```python
from build123d import *

# Parameters (mm, degrees)
EXTRUDE_1_DEPTH     = 50.5
EXTRUDE_2_DEPTH     = 4
CHAMFER_1_SIZE      = 10
SKETCH_3_R          = 4
CUT_EXTRUDE_1_DEPTH = 10
SKETCH_4_R          = 4
CUT_EXTRUDE_2_DEPTH = 10
SKETCH_5_R          = 2.5
CUT_EXTRUDE_3_DEPTH = 10


with BuildPart() as part:
    # 草图1 → 凸台-拉伸1 (new body)
    with BuildSketch(Plane.XY):
        Polygon((-12.426406871, 30), (-30, 12.426406871), (-30, -12.426406871), (-12.426406871, -30), (-12.426406871, -32.828427125), (-32, -13.254833996), (-32, 13.254833996), (-12.426406871, 32.828427125), align=None)
    extrude(amount=EXTRUDE_1_DEPTH)

    # 草图2 → 凸台-拉伸2 (add)
    with BuildSketch(Plane(origin=(0, 0, 0), x_dir=(-1, 0, 0), z_dir=(0, 0, -1))):
        Polygon((12.426406871, 30), (12.426406871, 40), (47.426406871, 40), (47.426406871, -40), (12.426406871, -40), (12.426406871, -30), (30, -12.426406871), (30, 12.426406871), align=None)
    extrude(amount=EXTRUDE_2_DEPTH)

    # 倒角1
    chamfer_1_edges = [part.edges().sort_by_distance(p)[0] for p in [
        (-47.426406871, -40, -2),
        (-47.426406871, 40, -2),
    ]]
    chamfer(chamfer_1_edges, length=CHAMFER_1_SIZE)

    # 草图3 → 切除-拉伸1 (cut)
    with BuildSketch(Plane(origin=(-22.627416998, 22.627416998, 0), x_dir=(0, 0, 1), z_dir=(-0.707106781, 0.707106781, 0))):
        with Locations((40.5, 0.585786438)):
            Circle(SKETCH_3_R)
        with Locations((24.5, 0.585786438)):
            Circle(SKETCH_3_R)
    cut_extrude_1 = extrude(amount=-CUT_EXTRUDE_1_DEPTH, mode=Mode.SUBTRACT)

    # 草图4 → 切除-拉伸2 (cut)
    with BuildSketch(Plane.ZY.offset(32)):
        with Locations((32.5, 0)):
            Circle(SKETCH_4_R)
    extrude(amount=-CUT_EXTRUDE_2_DEPTH, mode=Mode.SUBTRACT)

    # 镜向1: 切除-拉伸1 across plane
    add(cut_extrude_1.mirror(Plane.ZX), mode=Mode.SUBTRACT)

    # 草图5 → 切除-拉伸3 (cut)
    with BuildSketch(Plane.XY):
        with Locations((-38, 30)):
            Circle(SKETCH_5_R)
        with Locations((-38, -30)):
            Circle(SKETCH_5_R)
    extrude(amount=-CUT_EXTRUDE_3_DEPTH, mode=Mode.SUBTRACT)


solid = part.part
```
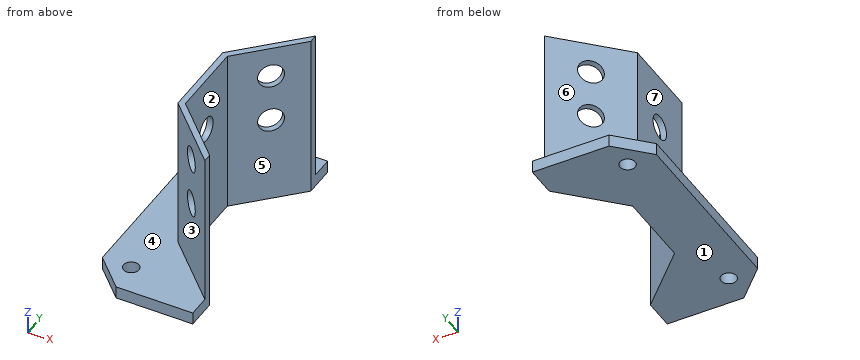
Model file for the job. Use its own axes, mm. Face numbers are marked on the shaded views. A direction names the side the tool comes from. Give positions to 0.01 mm unless a question says otherwise; leave off trailing zeros. Loops run counter-clockwise (first coordinate to the right, second up) from the corner with the lowest first, then second, coordinate; pieces in that order, holes last. Notation, with made-up numbers: (46, 9.25) -> (58, 9.25) arc R13 cw to (58, 13.25) -> close; hole circle Ø2 at (5.25, -13.5). An arc over 180 degrees is marked (long way). Write each question's results on one line, items separated by ' | '.
(1) Flat gauge pins, fed straight in: pin 1 Ø12 at (x, z) = (-24.5, 40) entering from -Y; pin 2 Ø13.5 at (y, z) = (-6, 30) entering from -X; pin 3 Ø6.5 at (x, y) = (-38, -30) entering from +Z. Where does each tip first touch, or does it go through?
Geometry results:
pin 1: stops at y = -26.75 | pin 2: stops at x = -32 | pin 3: stops at z = 0
(2) Pull direction Y, two halves, no side cores. Call the marked faces 1, 2 and 3: released by +Y, released by -Y, zero draft, split by the parting line, or undercut.
Geometry results:
face 1: zero draft | face 2: undercut | face 3: released by -Y
(3) Cut at C-C on z = 19. List the corners of the cut face in (x, y), and give its area (3 significant figures).
Geometry results:
outline: (-32, -13.25) -> (-12.43, -32.83) -> (-12.43, -30) -> (-30, -12.43) -> (-30, 12.43) -> (-12.43, 30) -> (-12.43, 32.83) -> (-32, 13.25) -> close | area: 156 mm²
(4) Cut at A-A on y = 0. List the corners of the cut face in (x, z).
Geometry results:
outline: (-47.43, -4) -> (-30, -4) -> (-30, 28.5) -> (-32, 28.5) -> (-32, 0) -> (-47.43, 0) -> close; (-32, 36.5) -> (-30, 36.5) -> (-30, 50.5) -> (-32, 50.5) -> close
(5) Cut at B-B on x = -38.5. List the corners of the cut face in (y, z), and give its area (3 significant figures).
Geometry results:
outline: (-38.93, -4) -> (-32.45, -4) -> (-32.45, 0) -> (-38.93, 0) -> close; (-27.55, -4) -> (27.55, -4) -> (27.55, 0) -> (-27.55, 0) -> close; (32.45, -4) -> (38.93, -4) -> (38.93, 0) -> (32.45, 0) -> close | area: 272 mm²
(6) Cut at D-D on z = 35.5. List the corners of the cut face in (x, y), and give its area (3 significant figures).
Geometry results:
outline: (-32, -13.25) -> (-12.43, -32.83) -> (-12.43, -30) -> (-30, -12.43) -> (-30, -2.65) -> (-32, -2.65) -> close; (-32, 2.65) -> (-30, 2.65) -> (-30, 12.43) -> (-12.43, 30) -> (-12.43, 32.83) -> (-32, 13.25) -> close | area: 146 mm²
(7) Probe line 1 along Y through (x, z) = (-38, -1); line 2 along Z through (x, y) = (-34.5, 8); line 3 along Y through (x, z) = (-31, 32). List the from-to ranges inside material, lowest first.
Geometry results:
line 1: y = -39.43 to -32.5, -27.5 to 27.5, 32.5 to 39.43 | line 2: z = -4 to 0 | line 3: y = -14.25 to -3.97, 3.97 to 14.25
(8) Tool access for the marked faces 4, 5, 6 and 7: list every direction of +Z, -Z, +X, -X, +Y, -Y with a clear straight run to the whole face (end or side of a thin tool).
Geometry results:
face 4: +Z, -X | face 5: +Z, -Z, +X | face 6: +Z, -X, +Y | face 7: +Z, -X, +Y, -Y
